Work out the finished part from the listing and answer in its coordinate system (mm). Coordinates: 2 decimals unless noted, no trailing zeros. Order: outer loops, then holes, each group sorted by start corner. A loop starts at its lowest first (then second) coordinate and runs counter-clockwise, first axis right, second up.
1. Flat-ended cylindrical pins translate along their axes: pin 1 Ø2 at (x, z) = (64, -9.5) entering from -Y; pin 2 Ø3 at (x, y) = (49, -5.5) entering from -Z. Find the tip coordinate at first contact, or state that the pin passes through.
2. The part is cut by section B-B, the plane x = 2. Give the vertices of the cut face in (y, z), then the cut area to 3 significant figures.
3. The part is cut by section A-A, the plane y = -4. Give the vertices of the cut face in (x, z), then the cut area to 3 significant figures.
4. Find the intervals of material crossed by probe 1 along Z at (x, y) = (-79, -5.25); probe 2 along Z at (x, y) = (-79, -4); probe 3 along Z at (x, y) = (-42.5, -1.5) (3 decimals), in increasing order.
```python
from build123d import *

# Parameters (mm, degrees)
BOSS_EXTRUDE1_DEPTH   = 83
M3X0_5_TAPPED_HOLE1_D = 2.5


with BuildPart() as part:
    # Sketch2 → Boss-Extrude1 (new body, symmetric)
    with BuildSketch(Plane(origin=(0, 0, 0), x_dir=(0, 0, -1), z_dir=(1, 0, 0))):
        Polygon((0, 0), (15.29, 0), (8.22, -7), (0, -7), align=None)
    extrude(amount=BOSS_EXTRUDE1_DEPTH, both=True)

    # M3x0.5 Tapped Hole1 (through all)
    with Locations(Plane(origin=(0, -7, 0), x_dir=(-1, 0, 0), z_dir=(0, -1, 0))):
        with Locations((79, 4), (-79, 4)):
            Hole(M3X0_5_TAPPED_HOLE1_D / 2)


solid = part.part
```
Geometry says:
1. pin 1: stops at y = -6.72
1. pin 2: stops at z = -11.25
2. outline: (-7, -8.22) - (0, -15.29) - (0, 0) - (-7, 0) - close
2. area: 82.3 mm2
3. outline: (-83, -11.25) - (83, -11.25) - (83, 0) - (-83, 0) - close; hole circle Ø2.5 at (-79, -4); hole circle Ø2.5 at (79, -4)
3. area: 1,860 mm2
4. probe 1: z = -9.99 to -5.25, -2.75 to 0
4. probe 2: z = -11.25 to -5.25, -2.75 to 0
4. probe 3: z = -13.775 to 0
